```python
from build123d import *

# Parameters (mm, degrees)
SKETCH_1_W               = 800
SKETCH_1_H               = 800
EXTRUDE_1_DEPTH          = 500
CUT_EXTRUDE_1_DEPTH      = 1025.695076596
CUT_EXTRUDE_1_DEPTH_BACK = 1025.695076596
CUT_EXTRUDE_2_DEPTH      = 1025.695076596
CUT_EXTRUDE_2_DEPTH_BACK = 1025.695076596


with BuildPart() as part:
    # 草图1 → 凸台-拉伸1 (new body)
    with BuildSketch(Plane(origin=(0, 0, 0), x_dir=(1, 0, 0), z_dir=(0, 1, 0))):
        Rectangle(SKETCH_1_W, SKETCH_1_H)
    extrude(amount=EXTRUDE_1_DEPTH)

    # 草图2 → 切除-拉伸1 (cut, two sides: drawn at the far end of the back side and taken through both)
    with BuildSketch(Plane.ZY.offset(400).offset(-CUT_EXTRUDE_1_DEPTH_BACK)):
        Polygon((-400, 240.192378865), (-250, 240.192378865), (-100, 500), (-400, 500), align=None)
        Polygon((250, 240.192378865), (100, 500), (400, 500), (400, 240.192378865), align=None)
    extrude(amount=CUT_EXTRUDE_1_DEPTH + CUT_EXTRUDE_1_DEPTH_BACK, mode=Mode.SUBTRACT)

    # 草图3 → 切除-拉伸2 (cut, two sides: drawn at the far end of the back side and taken through both)
    with BuildSketch(Plane(origin=(0, 0, -400), x_dir=(-1, 0, 0), z_dir=(0, 0, -1)).offset(-CUT_EXTRUDE_2_DEPTH_BACK)):
        Polygon((-400, 240.192378865), (-250, 240.192378865), (-100, 500), (-400, 500), align=None)
        Polygon((250, 240.192378865), (100, 500), (400, 500), (400, 240.192378865), align=None)
    extrude(amount=CUT_EXTRUDE_2_DEPTH + CUT_EXTRUDE_2_DEPTH_BACK, mode=Mode.SUBTRACT)


solid = part.part
```
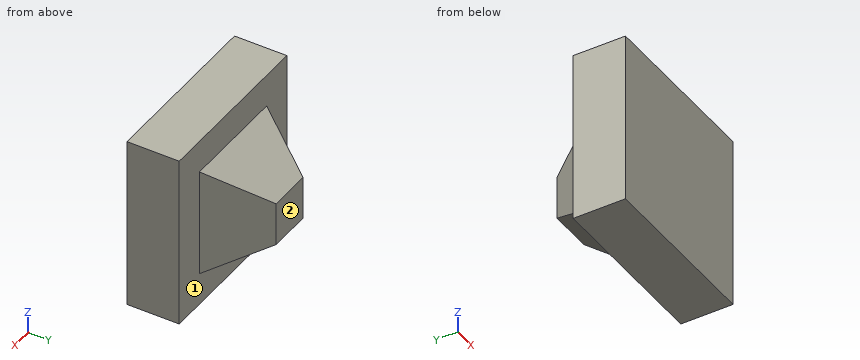
Check sheet for the modelled part. Datum: model origin and axes. Units: mm. Face numbers are marked on the shaded views. A direction names the side the tool comes from. Round coordinates to 2 decimals unless told otherwise and drop trailing zeros. Write each loop counter-clockwise with the first axis right and the second up, starting at its lowest first coordinate (ties: lowest second). Pieces come first, ordered by that corner, then holes. Notation, with made-up numbers: (38, 46) -> (80, 46) arc R27 cw to (80, 67) -> close; hole circle Ø3 at (-30.5, -9.75). An arc over 180 degrees is marked (long way). Put each result on its own line as item: value.
(1) Go/stop test with flat-tipped pins: pin 1 Ø3 at (x, z) = (-145.5, 13.5) entering from +Y; pin 2 Ø1 at (x, z) = (119.5, -110.5) entering from +Y. Record where each tip stops, or that it passes through.
Values found:
pin 1: stops at y = 423.79
pin 2: stops at y = 467.09
(2) Sectioned sample at C-C (y = 304). Enter the section's corners in (x, z), plus the area to 3 significant figures.
Values found:
outline: (-213.16, -213.16) -> (213.16, -213.16) -> (213.16, 213.16) -> (-213.16, 213.16) -> close
area: 182,000 mm^2
(3) Tool access check on the marked faces 1 and 2. Record the directions out of +Z, -Z, +X, -X, +Y, -Y that give a thin tool (end or side, any length) a straight path to the whole face; none if there is none.
Values found:
face 1: +Y
face 2: +Z, -Z, +X, -X, +Y
(4) Material ranges on line 1 (Y direction, x = 124, z = -322); line 2 (Z direction, x = 43, y = 319.5); line 3 (Z direction, x = 110.5, y = 297.5), recorded low to high.
Values found:
line 1: y = 0 to 240.19
line 2: z = -204.21 to 204.21
line 3: z = -216.91 to 216.91
(5) Sectioned sample at A-A (z = 27.5). Enter the section's corners in (x, y), plus the area to 3 significant figures.
Values found:
outline: (-400, 0) -> (400, 0) -> (400, 240.19) -> (250, 240.19) -> (100, 500) -> (-100, 500) -> (-250, 240.19) -> (-400, 240.19) -> close
area: 283,000 mm^2
(6) Sectioned sample at D-D (x = 307.5). Enter the section's corners in (y, z).
Values found:
outline: (0, -400) -> (240.19, -400) -> (240.19, 400) -> (0, 400) -> close
(7) Sectioned sample at B-B (x = 25). Enter the section's corners in (y, z).
Values found:
outline: (0, -400) -> (240.19, -400) -> (240.19, -250) -> (500, -100) -> (500, 100) -> (240.19, 250) -> (240.19, 400) -> (0, 400) -> close
